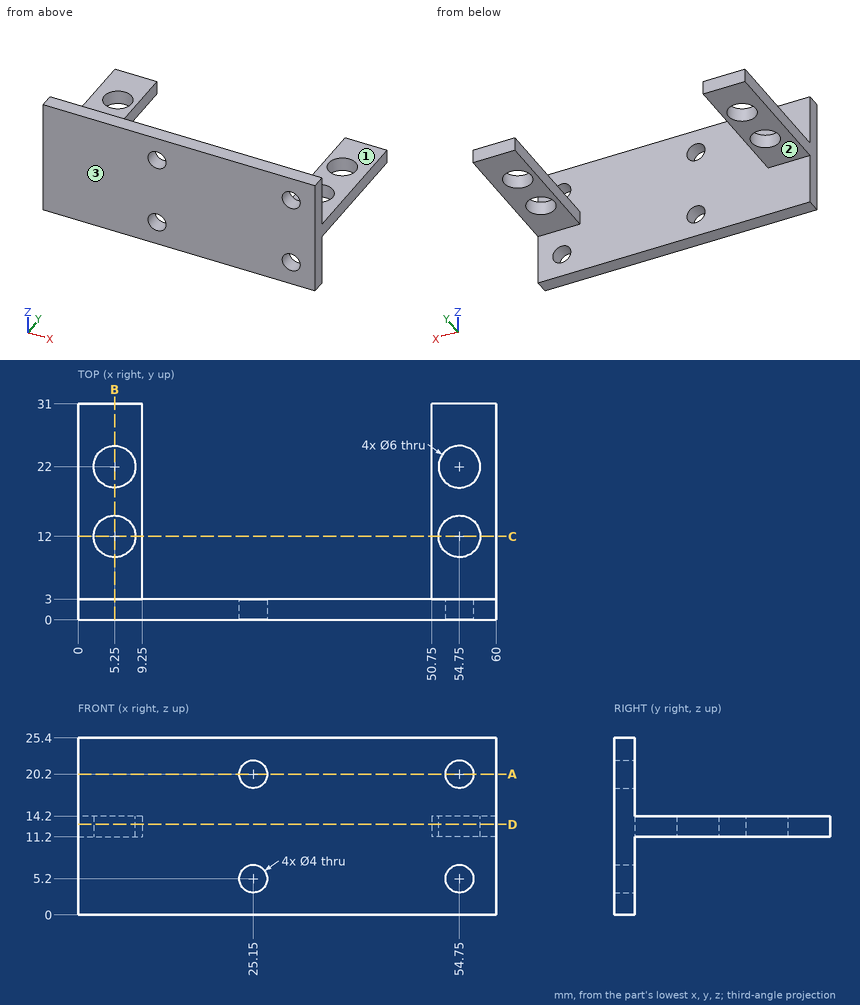
Answer from the drawing. Dimensions are ordinates in mm from the lowest x, y and z of the part. A direction names the side the tool comes from. Coordinates: 2 decimals unless noted, no trailing zeros. Write each loop counter-clockwise with the first axis right and the second up, starting at its lowest first coordinate (ties: lowest second). Pieces come first, ordered by that corner, then holes. Notation, with made-up numbers: (31.5, 35) - (57.5, 35) arc R10 ccw to (57.5, 47) - close; hole circle Ø11 at (88.25, 35). An arc over 180 degrees is marked (long way). Return JSON: item names as keys, results as strings.
1. The part is cut by section D-D on z = 13. Determine the outline of the cut face in (x, y).
Final values:
{"outline": "(0, 0) - (60, 0) - (60, 31) - (50.75, 31) - (50.75, 3) - (9.25, 3) - (9.25, 31) - (0, 31) - close; hole circle Ø6 at (5.25, 12); hole circle Ø6 at (5.25, 22); hole circle Ø6 at (54.75, 12); hole circle Ø6 at (54.75, 22)"}
2. Each of these flat-tipped pins is pushed along its axis until it touches: pin 1 Ø7.5 at (x, y) = (57, 22) entering from +Z; pin 2 Ø2 at (x, z) = (35, 17) entering from -Y; pin 3 Ø5 at (x, z) = (25.15, 5.2) entering from +Y; pin 4 Ø9.5 at (x, y) = (5.25, 12) entering from -Z. Where does it stop, or does it pass through?
Final values:
{"pin 1": "z = 14.2", "pin 2": "y = 0", "pin 3": "y = 3", "pin 4": "z = 11.2"}
3. The part is cut by section A-A on z = 20.2. Determine the outline of the cut face in (x, y).
Final values:
{"outline": "(0, 0) - (23.15, 0) - (23.15, 3) - (0, 3) - close; (27.15, 0) - (52.75, 0) - (52.75, 3) - (27.15, 3) - close; (56.75, 0) - (60, 0) - (60, 3) - (56.75, 3) - close"}
4. Which of the six approach directions +Z, -Z, +X, -X, +Y, -Y give full straight-line access (tool end or side, diameter ignored) to the marked faces 1, 2 and 3?
Final values:
{"face 1": "+Z, +X, -X, +Y", "face 2": "-Z, +X, -X, +Y", "face 3": "+Z, -Z, +X, -X, -Y"}
5. The part is cut by section B-B on x = 5.25. Determine the outline of the cut face in (y, z).
Final values:
{"outline": "(0, 0) - (3, 0) - (3, 11.2) - (9, 11.2) - (9, 14.2) - (3, 14.2) - (3, 25.4) - (0, 25.4) - close; (15, 11.2) - (19, 11.2) - (19, 14.2) - (15, 14.2) - close; (25, 11.2) - (31, 11.2) - (31, 14.2) - (25, 14.2) - close"}
6. Consider line 1 along X through (y, z) = (1.1, 5.2); line 2 along Z through (x, y) = (25.15, 1.4); line 3 along Y through (x, z) = (54.75, 11.9). Determine where each line is inside the solid, lowest interval first.
Final values:
{"line 1": "0 to 23.15, 27.15 to 52.75, 56.75 to 60", "line 2": "0 to 3.2, 7.2 to 18.2, 22.2 to 25.4", "line 3": "0 to 9, 15 to 19, 25 to 31"}
7. The part is cut by section C-C on y = 12. Determine the outline of the cut face in (x, z), then the cut area to 3 significant figures.
Final values:
{"outline": "(0, 11.2) - (2.25, 11.2) - (2.25, 14.2) - (0, 14.2) - close; (8.25, 11.2) - (9.25, 11.2) - (9.25, 14.2) - (8.25, 14.2) - close; (50.75, 11.2) - (51.75, 11.2) - (51.75, 14.2) - (50.75, 14.2) - close; (57.75, 11.2) - (60, 11.2) - (60, 14.2) - (57.75, 14.2) - close", "area": "19.5 mm^2"}
